Design review of the part built by this model. Coordinates are the model's own, in mm. A direction names the side the tool comes from. Round coordinates to 2 decimals unless told otherwise and drop trailing zeros. Order: outer loops, then holes, each group sorted by start corner. A loop starts at its lowest first (then second) coordinate and runs counter-clockwise, first axis right, second up. Notation, with made-up numbers: M 89,-21.5 L 132,-21.5 A23 ccw 132,4.5 Z; hole C -0.5,-7.5 d1. An arc over 180 degrees is marked long. Use a Markdown table: item, result. Add a question column.
(1) The part is to be moulded in two halves that separate along X. For faces 1 (the face through (227.81, 167.21, 20.36)), 2 (the face through (-273.05, 15, 20)), 3 (the face through (-268.221, 20.847, 25.395)), say which applies: released by +X, released by -X, zero draft, split by the parting line, or undercut.
(2) To check wall thickness, follow probe 1 along Y at (x, z) = (92, 27) (3 decimals); probe 2 along X at (y, z) = (105.5, 14.5); probe 3 along X at (y, z) = (224.5, 9). State the ranges of each line that lie inside material, in increasing order. Write a range as from..to.
(3) Take a section at C-C (x = -11). Write out the cut boundary in (y, z) (3 decimals).
(4) Take a section at B-B (y = 160). Write out the cut boundary in (x, z).
(5) Machinability: for faces 4 (the face through (-231.466, 179.369, 20.35)), 5 (the face through (110.211, 267.787, 20.922)), which of the approach directions +Z, -Z, +X, -X, +Y, -Y give a long, thin tool a straight path to every point of the face, cutting with its end or side? Answer none if there is none.
(6) Take a section at A-A (y = 225). Write out the cut boundary in (x, z), then the cut area to 3 significant figures.
(7) For pin 1 (4 mm diameter, centred on y = 176, z = 19.5, fed in from -X); pin 2 (5.5 mm diameter, centred on x = 53.98, z = 20.64, fed in from -Y); pin 3 (2 mm diameter, centred on x = -135.5, z = 5.5, fed in from -Y); pin 4 (3 mm diameter, centred on x = -98.5, z = 30.5, fed in from -Y), all flat-tipped, find the tip position at first contact; note any pin that passes through.
```python
from build123d import *

# Parameters (mm, degrees)
BOSS_EXTRUDE1_DEPTH = 41.275
SKETCH3_R           = 4.7625
CUT_EXTRUDE1_DEPTH  = 547.1
FILLET2_R           = 76.2
FILLET3_R           = 25.4
SKETCH7_R           = 3.175
CUT_EXTRUDE2_DEPTH  = 9.525


with BuildPart() as part:
    # Sketch2 → Boss-Extrude1 (new body)
    with BuildSketch(Plane.XY):
        with BuildLine():
            Line((-273.05, 0), (-273.05, 38.1))
            ThreePointArc((-273.05, 38.1), (-228.817032973, 183.397449758), (-111.125, 279.4))
            Line((-111.125, 279.4), (0, 279.4))
            Line((0, 279.4), (111.125, 279.4))
            ThreePointArc((111.125, 279.4), (228.817032973, 183.397449758), (273.05, 38.1))
            Line((273.05, 38.1), (273.05, 0))
            Line((273.05, 0), (263.525, 0))
            Line((263.525, 0), (263.525, 38.1))
            ThreePointArc((263.525, 38.1), (221.424095798, 177.317474829), (109.231868051, 269.875))
            Line((109.231868051, 269.875), (0, 269.875))
            Line((0, 269.875), (-109.231868051, 269.875))
            ThreePointArc((-109.231868051, 269.875), (-221.424095798, 177.317474829), (-263.525, 38.1))
            Line((-263.525, 38.1), (-263.525, 0))
            Line((-263.525, 0), (-273.05, 0))
        make_face()
    extrude(amount=BOSS_EXTRUDE1_DEPTH)

    # Sketch3 → Cut-Extrude1 (cut, through all)
    with BuildSketch(Plane(origin=(273.05, 0, 0), x_dir=(0, 0, -1), z_dir=(1, 0, 0))):
        with Locations((-20.6375, 20.6375)):
            Circle(SKETCH3_R)
        Polygon((0, 0), (-9.525, 0), (0, 279.4), align=None)
        Polygon((-31.75, 0), (-41.275, 279.4), (-41.275, 0), align=None)
    extrude(amount=-CUT_EXTRUDE1_DEPTH, mode=Mode.SUBTRACT)

    # Fillet2
    fillet2_edges = [part.edges().sort_by_distance(p)[0] for p in [
        (109.231868051, 269.875, 20.6375),
        (-109.231868051, 269.875, 20.6375),
    ]]
    fillet(fillet2_edges, radius=FILLET2_R)

    # Fillet3
    fillet3_edges = [part.edges().sort_by_distance(p)[0] for p in [
        (111.125, 279.4, 20.6375),
        (-111.125, 279.4, 20.6375),
    ]]
    fillet(fillet3_edges, radius=FILLET3_R)

    # Sketch7 → Cut-Extrude2 (cut)
    with BuildSketch(Plane(origin=(0, 279.4, 0), x_dir=(1, 0, 0), z_dir=(0, 1, 0))):
        with Locations((-53.975, -20.6375)):
            Circle(SKETCH7_R)
        with Locations((53.975, -20.6375)):
            Circle(SKETCH7_R)
    extrude(amount=-CUT_EXTRUDE2_DEPTH, mode=Mode.SUBTRACT)


solid = part.part
```
Verdict:
| question | item | result |
|---|---|---|
| 1 | face 1 | undercut |
| 1 | face 2 | released by -X |
| 1 | face 3 | zero draft |
| 2 | probe 1 | y = 269.875..279.4 |
| 2 | probe 2 | x = -264.19..-254.32, 254.32..264.19 |
| 2 | probe 3 | x = -194.64..-180.73, 180.73..194.64 |
| 3 | outline | M 269.875,0.325 L 279.4,0 L 279.4,41.275 L 269.875,40.95 Z |
| 4 | outline | M -242.8,4.07 L -231.97,4.07 L -231.97,37.2 L -242.8,37.2 Z; M 231.97,4.07 L 242.8,4.07 L 242.8,37.2 L 231.97,37.2 Z |
| 5 | face 4 | +Z, -Z, -X, +Y |
| 5 | face 5 | +Z, -Z, -Y |
| 6 | outline | M -194.12,1.85 L -180.18,1.85 L -180.18,39.42 L -194.12,39.42 Z; M 180.18,1.85 L 194.12,1.85 L 194.12,39.42 L 180.18,39.42 Z |
| 6 | area | 1,050 mm^2 |
| 7 | pin 1 | stops at x = -234.84 |
| 7 | pin 2 | passes through |
| 7 | pin 3 | stops at y = 256.48 |
| 7 | pin 4 | stops at y = 269.5 |
